from build123d import *

# Parameters (mm, degrees)
BASE_FLANGE1_DEPTH  = 102.87
CUT_EXTRUDE1_START  = -7.62
CUT_EXTRUDE1_DEPTH  = 7.62
SKETCH8_R           = 3.175
BOSS_EXTRUDE1_DEPTH = 3.81


# Read off the part's stored shape, not the designer's step: Cut-Extrude1
# Sheet-metal steps are written as plain solids
with BuildPart() as part:
    # Sketch2 → Base-Flange1 (new body)
    with BuildSketch(Plane(origin=(0, 0, 0), x_dir=(1, 0, 0), z_dir=(0, 1, 0))):
        with BuildLine():
            ThreePointArc((-119.38, 0), (45.684748156, 110.292738591), (84.414407538, -84.414407538))
            Line((84.414407538, -84.414407538), (83.893552683, -83.893552683))
            ThreePointArc((83.893552683, -83.893552683), (45.402863539, 109.612208928), (-118.6434, 0))
            Line((-118.6434, 0), (-119.38, 0))
        make_face()
    extrude(amount=BASE_FLANGE1_DEPTH)

    # Cut-Extrude1 outline → Cut-Extrude1 (cut)
    with BuildSketch(Plane.XZ.offset(CUT_EXTRUDE1_START)):
        with BuildLine():
            ThreePointArc((-119.38, 0), (28.374941826, -115.958816294), (105.891353265, 55.123549448))
            Line((105.891353265, 55.123549448), (105.237981085, 54.783425419))
            ThreePointArc((105.237981085, 54.783425419), (28.199862397, -115.243325726), (-118.6434, 0))
            Line((-118.6434, 0), (-119.38, 0))
        make_face()
    extrude(amount=CUT_EXTRUDE1_DEPTH, mode=Mode.SUBTRACT)

    # Sketch8 → Boss-Extrude1 (add)
    with BuildSketch(Plane.XZ):
        with BuildLine():
            Line((105.891353265, 55.123549448), (124.635571409, 69.054164544))
            ThreePointArc((124.635571409, 69.054164544), (123.499250093, 84.844358217), (108.336377108, 89.39504225))
            Line((108.336377108, 89.39504225), (84.414407538, 84.414407538))
            ThreePointArc((84.414407538, 84.414407538), (96.273356857, 70.590545822), (105.891353265, 55.123549448))
        make_face()
        with Locations(Location((112.618181959, 76.125332112, 0), (0, 0, 270))):
            Circle(SKETCH8_R, mode=Mode.SUBTRACT)
    extrude(amount=-BOSS_EXTRUDE1_DEPTH)


solid = part.part
Geometry: final body of the model. Coordinates: model frame, mm. Give positions to 0.01 mm unless a question says otherwise; leave off trailing zeros. Write each loop counter-clockwise with the first axis right and the second up, starting at its lowest first coordinate (ties: lowest second). Pieces come first, ordered by that corner, then holes. Notation, with made-up numbers: (-16, 53.25) - (-9, 53.25) arc R28 ccw to (-9, 79.25) - close; hole circle Ø1 at (37, 1). An arc over 180 degrees is marked (long way). Return JSON: item names as keys, results as strings. Group by question number.
1) First-contact query: P1, Ø10.5, axis at x = 109.5, z = 70.5, coming from the +Y side; P2, Ø2, axis at x = 35.5, y = 68, coming from the +Z side; P3, Ø12, axis at y = 19.5, z = 67.5, coming from the +X side; P4, Ø4, axis at x = 112.62, z = 76.13, coming from the +Y side. Flat tips, straight axial feed; report the tip coordinate or a pass-through.
2) Section B-B on x = 0. Return the cut outline in (y, z), plus the area to 3 significant figures.
3) Section A-A on z = -15. Return the cut outline in (x, y).
4) Line query: line 1 (Z direction, x = 0, y = 54); line 2 (X direction, y = 36, z = -68); line 3 (X direction, y = 49.5, z = -96.5). Output: solid intervals per line, ascending.
5) Mould query, pull axis Z, two halves, no side actions, for faces 1 (the cylindrical face through (109.519, 1.878, 76.814)), 2 (the flat face through (110, 3.81, 73)), 3 (the cylindrical face through (42.636, 52.647, -111.507)). Classes: released by +Z, released by -Z, zero draft, split by the parting line, or undercut.
6) Section D-D on z = -41.5. Return the cut outline in (x, y), plus the area to 3 significant figures.
7) Section C-C on y = 31. Return the cut outline in (x, z).
Filled in:
{
 "1": {"P1": "stops at y = 3.81", "P2": "stops at z = -112.89", "P3": "stops at x = 102.32", "P4": "passes through"},
 "2": {"outline": "(7.62, -119.38) - (102.87, -119.38) - (102.87, -118.64) - (7.62, -118.64) - close", "area": "70.2 mm^2"},
 "3": {"outline": "(-118.43, 7.62) - (-117.69, 7.62) - (-117.69, 102.87) - (-118.43, 102.87) - close; (117.69, 7.62) - (118.43, 7.62) - (118.43, 102.87) - (117.69, 102.87) - close"},
 "4": {"line 1": "z = -119.38 to -118.64", "line 2": "x = -98.12 to -97.22, 97.22 to 98.12", "line 3": "x = -70.28 to -69.02, 69.02 to 70.28"},
 "5": {"face 1": "undercut", "face 2": "zero draft", "face 3": "split by the parting line"},
 "6": {"outline": "(-111.93, 7.62) - (-111.15, 7.62) - (-111.15, 102.87) - (-111.93, 102.87) - close; (111.15, 7.62) - (111.93, 7.62) - (111.93, 102.87) - (111.15, 102.87) - close", "area": "150 mm^2"},
 "7": {"outline": "(-119.38, 0) arc R119.38 ccw (long way) to (84.41, 84.41) - (83.89, 83.89) arc R118.64 cw (long way) to (-118.64, 0) - close"}
}
